from build123d import *

# Parameters (mm, degrees)
SKETCH3_R           = 3.175
BOSS_EXTRUDE1_DEPTH = 3.175


with BuildPart() as part:
    # Sketch3 → Boss-Extrude1 (new body)
    with BuildSketch(Plane.XY):
        Polygon((76.2, 0), (-76.2, 0), (-101.6, -25.4), (101.6, -25.4), align=None)
        with Locations((-69.85, -12.7)):
            Circle(SKETCH3_R, mode=Mode.SUBTRACT)
        with Locations(Location((69.85, -12.7, 0), (0, 0, 180))):
            Circle(SKETCH3_R, mode=Mode.SUBTRACT)
    extrude(amount=BOSS_EXTRUDE1_DEPTH)


solid = part.part
Geometry check sheet. Reference: the model listing, model coordinates, mm. Round coordinates to 2 decimals unless told otherwise and drop trailing zeros. Order: outer loops, then holes, each group sorted by start corner. A loop starts at its lowest first (then second) coordinate and runs counter-clockwise, first axis right, second up. Notation, with made-up numbers: M -25,80 L -9,80 A19 cw -9,104 Z; hole C 89,44.5 d3. An arc over 180 degrees is marked long. Write each question's results on one line, items separated by ' | '. Start each with the question number.
1. Cross-section at D-D on y = -23.25. Record the boundary of the cut face in (x, z) (3 decimals), plus the area to 3 significant figures.
2. Cross-section at B-B on y = -12.7. Record the boundary of the cut face in (x, z) (3 decimals).
3. Cross-section at C-C on z = 2.15. Record the boundary of the cut face in (x, y) (3 decimals), plus the area to 3 significant figures.
4. Go/stop test with flat-tipped pins: P1, Ø5, axis at x = -69.85, y = -12.7, coming from the +Z side; P2, Ø1, axis at y = -3.5, z = 1, coming from the +X side. Record where each tip stops, or that it passes through.
5. Material ranges on L1, parallel to Y at x = 69.85, z = 1.1 (3 decimals); L2, parallel to X at y = -13.5, z = 1.2; L3, parallel to X at y = -18.75, z = 1.9, recorded low to high. Write a range as from..to.
6. Draft check along X on faces 1 (the face through (1, 0, 2)), 2 (the face through (72.37, -10.77, 1.57)), 3 (the face through (-88.7, -12.5, 1.6)), 4 (the face through (89.1, -12.9, 1.6)). Enter one of: pulls with the +X half, pulls with the -X half, needs draft (parallel to the pull), parting line crosses it, or undercut.
7. Cross-section at A-A on x = -69.85. Record the boundary of the cut face in (y, z) (3 decimals).
Resolved:
1) outline: M -99.45,0 L 99.45,0 L 99.45,3.175 L -99.45,3.175 Z | area: 632 mm2
2) outline: M -88.9,0 L -73.025,0 L -73.025,3.175 L -88.9,3.175 Z; M -66.675,0 L 66.675,0 L 66.675,3.175 L -66.675,3.175 Z; M 73.025,0 L 88.9,0 L 88.9,3.175 L 73.025,3.175 Z
3) outline: M -101.6,-25.4 L 101.6,-25.4 L 76.2,0 L -76.2,0 Z; hole C -69.85,-12.7 d6.35; hole C 69.85,-12.7 d6.35 | area: 4,450 mm2
4) P1: through | P2: x = 80.2
5) L1: -25.4..-15.875, -9.525..0 | L2: -89.7..-72.92, -66.78..66.78, 72.92..89.7 | L3: -94.95..94.95
6) face 1: needs draft | face 2: undercut | face 3: pulls with the -X half | face 4: pulls with the +X half
7) outline: M -25.4,0 L -15.875,0 L -15.875,3.175 L -25.4,3.175 Z; M -9.525,0 L 0,0 L 0,3.175 L -9.525,3.175 Z
